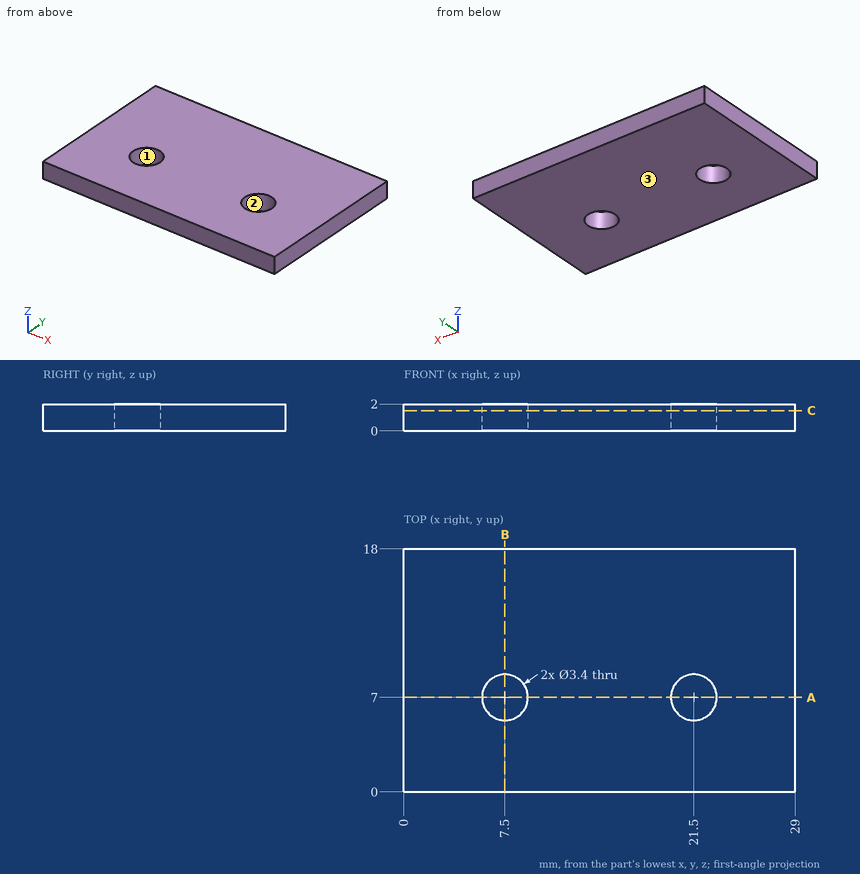
Input: dimensioned drawing with shaded views. Units: mm. Origin: part minimum x, y, z. Give positions to 0.01 mm unless a question says otherwise; leave off trailing zeros. Write each loop counter-clockwise with the first axis right and the second up, starting at its lowest first coordinate (ties: lowest second). Pieces come first, ordered by that corner, then holes. Notation, with made-up numbers: (-4, -23) -> (37, -23) arc R19 cw to (37, 6) -> close; hole circle Ø10 at (28, -18.5). An arc over 180 degrees is marked (long way). Answer as a JSON object with one key per item and string values.
1. Ray query, probe 1 along Y at (x, z) = (7.5, 1.15); probe 2 along X at (y, z) = (8.25, 1.4); probe 3 along X at (y, z) = (8.5, 1). Return the intervals inside material, ascending. Write a range as from..to.
Ans:
{"probe 1": "y = 0..5.3, 8.7..18", "probe 2": "x = 0..6.35, 8.65..20.35, 22.65..29", "probe 3": "x = 0..6.7, 8.3..20.7, 22.3..29"}
2. Cut plane B-B on x = 7.5. Output: boundary loops of the cut face in (y, z).
Ans:
{"outline": "(0, 0) -> (5.3, 0) -> (5.3, 2) -> (0, 2) -> close; (8.7, 0) -> (18, 0) -> (18, 2) -> (8.7, 2) -> close"}
3. Cut plane C-C on z = 1.5. Output: boundary loops of the cut face in (x, y).
Ans:
{"outline": "(0, 0) -> (29, 0) -> (29, 18) -> (0, 18) -> close; hole circle Ø3.4 at (7.5, 7); hole circle Ø3.4 at (21.5, 7)"}
4. Cut plane A-A on y = 7. Output: boundary loops of the cut face in (x, z).
Ans:
{"outline": "(0, 0) -> (5.8, 0) -> (5.8, 2) -> (0, 2) -> close; (9.2, 0) -> (19.8, 0) -> (19.8, 2) -> (9.2, 2) -> close; (23.2, 0) -> (29, 0) -> (29, 2) -> (23.2, 2) -> close"}
5. Mould query, pull axis Y, two halves, no side actions, for the marked faces 1, 2 and 3. Classes: pulls with the +Y half, pulls with the -Y half, needs draft (parallel to the pull), parting line crosses it, or undercut.
Ans:
{"face 1": "undercut", "face 2": "undercut", "face 3": "needs draft"}
